Could you check a few things on this model? Use its own coordinates, in mm. Give positions to 0.01 mm unless a question says otherwise; leave off trailing zeros. Loops run counter-clockwise (first coordinate to the right, second up) from the corner with the lowest first, then second, coordinate; pieces in that order, holes last. Notation, with made-up numbers: (69, -32.5) - (92, -32.5) arc R20 ccw to (92, 6.5) - close; hole circle Ø10 at (70.5, -33). An arc over 180 degrees is marked (long way). One line per item, written item: value. Start each with the question number.
Q1. I'm going to push flat-ended pins straight in: P1, Ø10, axis at x = 13, y = -2.5, coming from the +Z side; P2, Ø1.5, axis at x = -2.5, y = -4, coming from the +Z side; P3, Ø1, axis at x = 10, y = 5.5, coming from the -Z side; P4, Ø16, axis at x = 0, z = 0, coming from the -Y side. Where does each tip first touch, or does it pass through?
Q2. If I drill on line 1 (X direction, y = -5.75, z = 0); line 2 (Z direction, x = 1, y = 9); line 3 (X direction, y = 9.5, z = -1.5), over which ranges is the centre line in solid material (lowest first)? Write a range as from..to.
Q3. If we mould it in two halves opening along X, with no side actions, what happens to faces 1 (the face through (-2.703, -5.07, -8.584)), 2 (the face through (7, 11.229, 18)), 3 (the face through (-2.83, 0.64, -9)), 4 (the face through (10.74, -5.24, 2.38))? For each: released by +X, released by -X, zero draft, split by the parting line, or undercut.
Q4. I want a section at C-C (y = 7). Please give me the cut outline in (x, z).
Q5. I want a section at D-D (y = -3). Please give me the cut outline in (x, z), then the cut area to 3 significant figures.
Q6. I want a section at A-A (z = 0). Please give me the cut outline in (x, y), then the cut area to 3 significant figures.
Q7. I want a section at B-B (x = 0). Please give me the cut outline in (y, z).
```python
from build123d import *


with BuildPart() as part:
    # Sketch1 → Revolve-Thin3 (revolve)
    with BuildSketch(Plane.XY, mode=Mode.PRIVATE) as revolve_thin3_sk:
        Polygon((-20, 13.228756555), (-18, 13.228756555), (-9, 0), (-9, -10), (-11, -10), (-11, -0.615831877), (-19.058300524, 11.228756555), (-20, 11.228756555), align=None)
    revolve(revolve_thin3_sk.sketch.rotate(Axis((0, 0, 0), (0, 1, 0)), 270), axis=Axis((0, 0, 0), (0, 1, 0)))


solid = part.part
```
Worked answers:
1. P1: stops at z = 7.59
1. P2: stops at z = 10.86
1. P3: stops at z = -12.01
1. P4: passes through
2. line 1: x = -11..-9, 9..11
2. line 2: z = -17.51..-15.09, 15.09..17.51
2. line 3: x = -17.82..-15.39, 15.39..17.82
3. face 1: undercut
3. face 2: zero draft
3. face 3: undercut
3. face 4: split by the parting line
4. outline: circle Ø32.36 at (0, 0); hole circle Ø27.52 at (0, 0)
5. outline: circle Ø22 at (0, 0); hole circle Ø18 at (0, 0)
5. area: 126 mm²
6. outline: (-20, 11.23) - (-19.06, 11.23) - (-11, -0.62) - (-11, -10) - (-9, -10) - (-9, 0) - (-18, 13.23) - (-20, 13.23) - close; (9, -10) - (11, -10) - (11, -0.62) - (19.06, 11.23) - (20, 11.23) - (20, 13.23) - (18, 13.23) - (9, 0) - close
6. area: 105 mm²
7. outline: (-10, -11) - (-0.62, -11) - (11.23, -19.06) - (11.23, -20) - (13.23, -20) - (13.23, -18) - (0, -9) - (-10, -9) - close; (-10, 9) - (0, 9) - (13.23, 18) - (13.23, 20) - (11.23, 20) - (11.23, 19.06) - (-0.62, 11) - (-10, 11) - close
